Design review of the part built by this model. Coordinates are the model's own, in mm. Face numbers are marked on the shaded views. A direction names the side the tool comes from. Coordinates: 2 decimals unless noted, no trailing zeros. Write each loop counter-clockwise with the first axis right and the second up, starting at its lowest first coordinate (ties: lowest second). Pieces come first, ordered by that corner, then holes. Notation, with made-up numbers: (88.5, -14.75) - (136.5, -14.75) arc R26 ccw to (136.5, 4.25) - close; hole circle Ø6 at (51.25, -31). An arc over 180 degrees is marked (long way). Use a Markdown table: item, result.
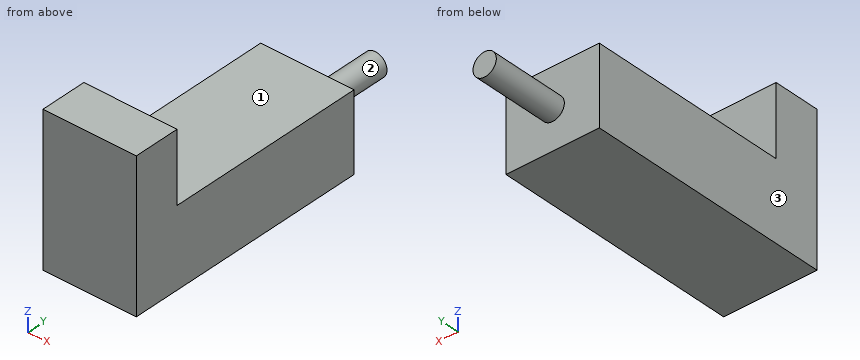
from build123d import *

# Parameters (mm, degrees)
SKETCH_1_W      = 12
SKETCH_1_H      = 10
EXTRUDE_1_DEPTH = 32
SKETCH_2_R      = 1.5
EXTRUDE_2_DEPTH = 10
SKETCH_3_W      = 12
SKETCH_3_H      = 6
EXTRUDE_3_DEPTH = 9


with BuildPart() as part:
    # 草图1 → 凸台-拉伸1 (new body)
    with BuildSketch(Plane(origin=(0, 0, 0), x_dir=(1, 0, 0), z_dir=(0, 1, 0))):
        Rectangle(SKETCH_1_W, SKETCH_1_H)
    extrude(amount=EXTRUDE_1_DEPTH)

    # 草图2 → 凸台-拉伸2 (add)
    with BuildSketch(Plane(origin=(0, 32, 0), x_dir=(1, 0, 0), z_dir=(0, 1, 0))):
        with Locations(Location((0, 0, 0), (0, 0, 270))):
            Circle(SKETCH_2_R)
    extrude(amount=EXTRUDE_2_DEPTH)

    # 草图3 → 凸台-拉伸3 (add)
    with BuildSketch(Plane.XY.offset(5)):
        with Locations((0, 3)):
            Rectangle(SKETCH_3_W, SKETCH_3_H)
    extrude(amount=EXTRUDE_3_DEPTH)


solid = part.part
(1) Take a section at A-A on x = 0. Write out the cut boundary in (y, z), and give its area (3 significant figures).
Determined:
| item | result |
|---|---|
| outline | (0, -5) - (32, -5) - (32, -1.5) - (42, -1.5) - (42, 1.5) - (32, 1.5) - (32, 5) - (6, 5) - (6, 14) - (0, 14) - close |
| area | 404 mm2 |
(2) Take a section at D-D on z = 2. Write out the cut boundary in (x, y).
Determined:
| item | result |
|---|---|
| outline | (-6, 0) - (6, 0) - (6, 32) - (-6, 32) - close |
(3) Take a section at B-B on z = 0. Write out the cut boundary in (x, y), and give its area (3 significant figures).
Determined:
| item | result |
|---|---|
| outline | (-6, 0) - (6, 0) - (6, 32) - (1.5, 32) - (1.5, 42) - (-1.5, 42) - (-1.5, 32) - (-6, 32) - close |
| area | 414 mm2 |
(4) For L1, parallel to Z at x = -2, y = 9; L2, parallel to Y at x = -3, z = -1; L3, parallel to Y at x = -3.75, z = 12.5, list the stretches that pass through material, from the lowest coordinate up. Write a range as from..to.
Determined:
| item | result |
|---|---|
| L1 | -5..5 |
| L2 | 0..32 |
| L3 | 0..6 |
(5) Machinability: for the marked faces 1, 2 and 3, which of the approach directions +Z, -Z, +X, -X, +Y, -Y give a long, thin tool a straight path to every point of the face, cutting with its end or side? Answer none if there is none.
Determined:
| item | result |
|---|---|
| face 1 | +Z, +X, -X, +Y |
| face 2 | +Y |
| face 3 | +Z, -Z, -X, +Y, -Y |
(6) Take a section at C-C on y = 37. Write out the cut boundary in (x, z), and give its area (3 significant figures).
Determined:
| item | result |
|---|---|
| outline | circle Ø3 at (0, 0) |
| area | 7.07 mm2 |
(7) For pin 1 (6 mm diameter, centred on x = -1.5, y = 24.5, fed in from +Z); pin 2 (1 mm diameter, centred on y = 16.5, z = 6, fed in from -X); pin 3 (1.5 mm diameter, centred on x = -3.5, z = 12, fed in from +Y), all flat-tipped, find the tip position at first contact; note any pin that passes through.
Determined:
| item | result |
|---|---|
| pin 1 | z = 5 |
| pin 2 | through |
| pin 3 | y = 6 |
